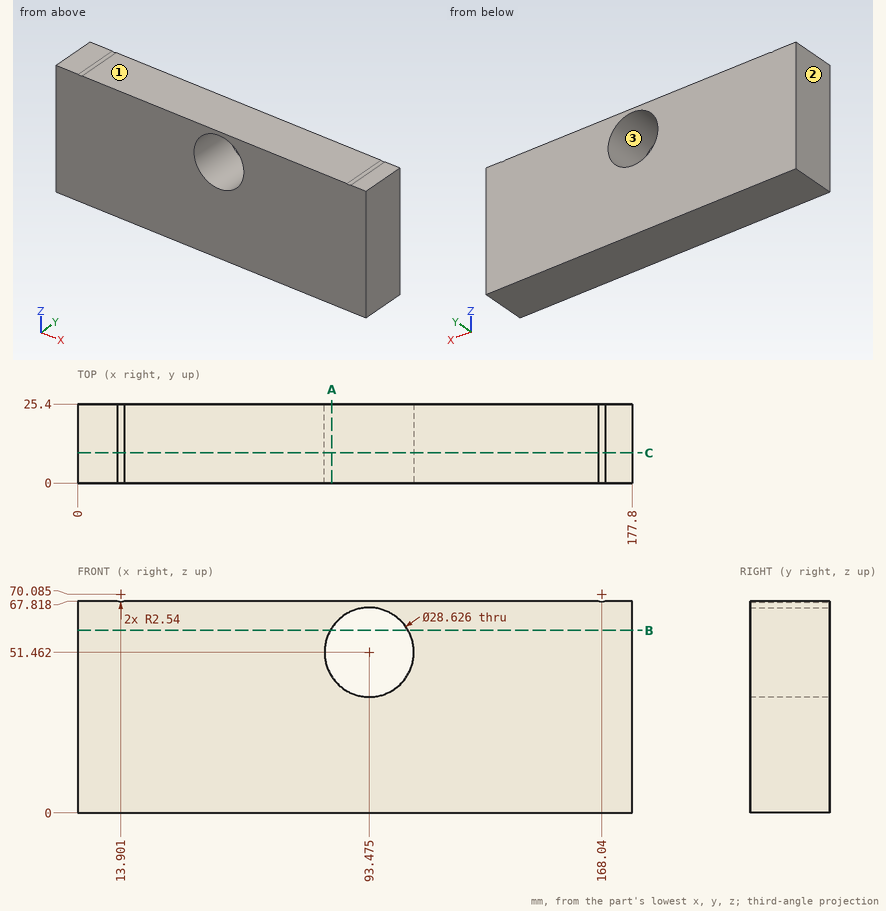
Here's the drawing with two shaded views (mm, measured from the low corner). I have some questions. Round coordinates to 2 decimals unless told otherwise and drop trailing zeros. Loops run counter-clockwise (first coordinate to the right, second up) from the corner with the lowest first, then second, coordinate; pieces in that order, holes last.
Item 1: If we mould it in two halves opening along X, with no side actions, what happens to the marked faces 1, 2 and 3? For each: +X half, -X half, draft (parallel to the pull), parting line (faces both ways), or undercut.
Item 2: Please list where these lines run through material, in increasing order: L1, parallel to X at y = 14, z = 49 (1 decimal); L2, parallel to X at y = 21.25, z = 40 (1 decimal); L3, parallel to Z at x = 99, y = 22.5 (1 decimal).
Item 3: Suppose I cut it at B-B, the plane z = 58.5. Write out the boundary of the cut face in (x, y), then the cut area to 3 significant figures.
Item 4: Suppose I cut it at C-C, the plane y = 9.75. Write out the boundary of the cut face in (x, z) (1 decimal).
Item 5: Will this pin go through, and if not, where does the flat tip stop? pin 1 Ø10 at (x, y) = (50.5, 13.5) entering from -Z.
Item 6: Suppose I cut it at A-A, the plane x = 81.5. Write out the boundary of the cut face in (y, z), then the cut area to 3 significant figures.
Reported:
1. face 1: draft
1. face 2: -X half
1. face 3: undercut
2. L1: x = 0 to 79.4, 107.6 to 177.8
2. L2: x = 0 to 84.9, 102 to 177.8
2. L3: z = 0 to 38.3, 64.7 to 67.8
3. outline: (0, 0) - (81.01, 0) - (81.01, 25.4) - (0, 25.4) - close; (105.94, 0) - (177.8, 0) - (177.8, 25.4) - (105.94, 25.4) - close
3. area: 3,880 mm2
4. outline: (0, 0) - (177.8, 0) - (177.8, 67.8) - (169.2, 67.8) arc R2.5 cw to (166.9, 67.8) - (15, 67.8) arc R2.5 cw to (12.8, 67.8) - (0, 67.8) - close; hole circle Ø28.6 at (93.5, 51.5)
5. pin 1: stops at z = 0
6. outline: (0, 0) - (25.4, 0) - (25.4, 43.62) - (0, 43.62) - close; (0, 59.3) - (25.4, 59.3) - (25.4, 67.82) - (0, 67.82) - close
6. area: 1,320 mm2
